Answer from the drawing. Dimensions are ordinates in mm from the lowest x, y and z of the part. A direction names the side the tool comes from. Round coordinates to 2 decimals unless told otherwise and drop trailing zeros. Loops run counter-clockwise (first coordinate to the right, second up) from the corner with the lowest first, then second, coordinate; pieces in that order, holes last. Notation, with made-up numbers: (39, 78) - (68, 78) arc R21 ccw to (68, 115) - close; hole circle Ø9 at (6.25, -31.5). An arc over 180 degrees is marked (long way). Return JSON: item names as keys, results as strings.
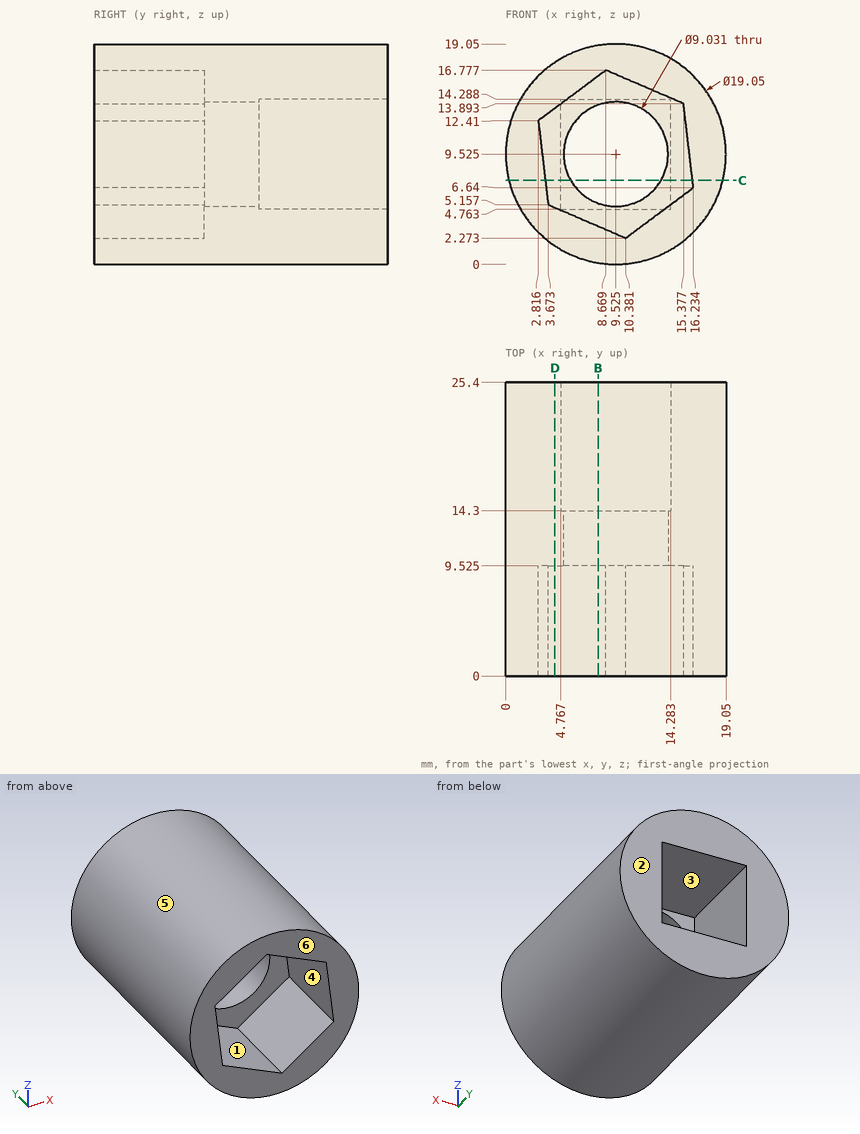
1) A tool of negligible diameter and unlimited length cuts with its end or side. For the marked faces 1, 2 and 3, from which of +Z, -Z, +X, -X, +Y, -Y can it reach the whole face along a straight path? Write none if from no direction.
Verdict:
{"face 1": "-Y", "face 2": "+Z, -Z, +X, -X, +Y", "face 3": "+Y"}
2) Section B-B (x = 8) is taken. Give the vertices of the cut face in (y, z) (1 decimal).
Verdict:
{"outline": "(0, 0.1) - (25.4, 0.1) - (25.4, 4.8) - (14.3, 4.8) - (14.3, 5.3) - (9.5, 5.3) - (9.5, 3.3) - (0, 3.3) - close; (0, 16.3) - (9.5, 16.3) - (9.5, 13.8) - (14.3, 13.8) - (14.3, 14.3) - (25.4, 14.3) - (25.4, 18.9) - (0, 18.9) - close"}
3) Find the intervals of material crossed by L1, parallel to Y at x = 10, z = 4.25 (1 decimal); L2, parallel to Z at x = 12.75, y = 16.25; L3, parallel to Z at x = 8.75, y = 21.25, in increasing order.
Verdict:
{"L1": "y = 9.5 to 25.4", "L2": "z = 0.56 to 4.76, 14.29 to 18.49", "L3": "z = 0.03 to 4.76, 14.29 to 19.02"}
4) Flat-ended cylindrical pins translate along their axes: pin 1 (1 mm diameter, centred on y = 4, z = 12, fed in from +X); pin 2 (10.5 mm diameter, centred on x = 9.5, z = 8.5, fed in from +Y); pin 3 (1.5 mm diameter, centred on x = 2.5, y = 4, fed in from +Z); pin 4 (10.5 mm diameter, centred on x = 9.5, z = 10.5, fed in from -Y) (1 decimal). Find the tip coordinate at first contact, or state that the pin passes through.
Verdict:
{"pin 1": "stops at x = 18.84", "pin 2": "stops at y = 25.4", "pin 3": "stops at z = 16.69", "pin 4": "stops at y = 9.5"}
5) Section D-D (x = 4.25) is taken. Give the vertices of the cut face in (y, z) (1 decimal), and give its area (3 significant figures).
Verdict:
{"outline": "(0, 1.6) - (25.4, 1.6) - (25.4, 17.5) - (0, 17.5) - (0, 13.5) - (9.5, 13.5) - (9.5, 4.9) - (0, 4.9) - close", "area": "321 mm2"}
6) Section C-C (z = 7.25) is taken. Give the vertices of the cut face in (x, y) (1 decimal), and give its area (3 significant figures).
Verdict:
{"outline": "(0.3, 0) - (3.4, 0) - (3.4, 9.5) - (5.6, 9.5) - (5.6, 14.3) - (4.8, 14.3) - (4.8, 25.4) - (0.3, 25.4) - close; (13.4, 9.5) - (16.2, 9.5) - (16.2, 0) - (18.8, 0) - (18.8, 25.4) - (14.3, 25.4) - (14.3, 14.3) - (13.4, 14.3) - close", "area": "206 mm2"}
7) Determine the mould class of the marked faces 4, 5 and 6 for opening direction Z: pulls with the +Z half, pulls with the -Z half, needs draft (parallel to the pull), parting line crosses it, or undercut.
Verdict:
{"face 4": "undercut", "face 5": "parting line crosses it", "face 6": "needs draft"}
